Work out the finished part from the listing and answer in its coordinate system (mm). Face numbers are marked on the shaded views. A direction names the side the tool comes from. Give positions to 0.01 mm unless a question says otherwise; leave off trailing zeros. Write each loop counter-clockwise with the first axis right and the second up, starting at its lowest first coordinate (ties: lowest second). Pieces come first, ordered by that corner, then holes.
1) Given pin 1 Ø2 at (x, z) = (50, 44) entering from -Y; pin 2 Ø5 at (x, z) = (14, 6.5) entering from +Y; pin 3 Ø1.6 at (x, y) = (39, 110) entering from -Z; pin 4 Ø10 at (y, z) = (75.5, 37.5) entering from -X, each flat-ended and moving along its own axis, determine where each tip first touches the part or whether it passes through.
2) Find section A-A (y = 30). Determine the outline of the cut face in (x, z).
3) Find section B-B (x = 37). Count the separate pieces of the cut face and the enclosed holes in it, plus the area to 3 significant figures.
4) Determine the mould class of the marked faces 4, 5, 6 and 7 for opening direction Z: pulls with the +Z half, pulls with the -Z half, needs draft (parallel to the pull), parting line crosses it, or undercut.
5) A tool of negligible diameter and unlimited length cuts with its end or side. For the marked faces 1, 2 and 3, from which of +Z, -Z, +X, -X, +Y, -Y can it reach the whole face along a straight path? Write none if from no direction.
6) Straight lines are drawn through the part: probe 1 along Y at (x, z) = (55.5, 25.4); probe 2 along X at (y, z) = (11.5, 41); probe 3 along Z at (x, y) = (53, 107.5). For each, find the intervals that lie inside material, in ascending order.
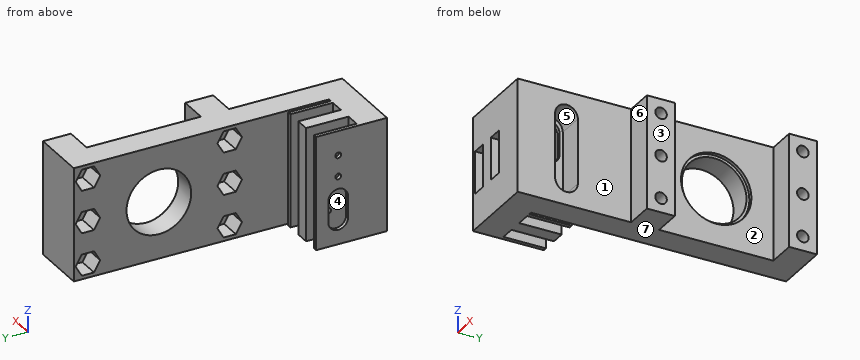
Autodesk Inventor part; units mm, degrees
ref_plane "YZ Plane" through (0, 0, 0) normal (1, 0, 0) x (0, 1, 0)
ref_plane "XZ Plane" through (0, 0, 0) normal (0, 1, 0) x (-1, 0, 0)
ref_plane "XY Plane" through (0, 0, 0) normal (0, 0, 1) x (1, 0, 0)
sketch "Sketch1" plane through (0, 0, 0) normal (0, 0, 1) x (1, 0, 0)
  line L0 (10.0241, 20.4474) -> (11.6941, 20.4474)
  line L1 (11.6941, 20.4474) -> (11.6941, -11.3026)
  line L2 (11.6941, -11.3026) -> (10.0241, -11.3026)
  line L3 (10.0241, -11.3026) -> (10.0241, 20.4474)
  line L4 (11.6941, -4.9526) -> (18.1941, -4.9526)
  line L5 (18.1941, -4.9526) -> (18.1941, -11.3026)
  line L6 (18.1941, -11.3026) -> (11.6941, -11.3026)
  line L7 (11.6941, -11.3026) -> (11.6941, -4.9526)
  line L8 (18.1941, 20.4474) -> (24.3941, 20.4474)
  line L9 (24.3941, 20.4474) -> (24.3941, -11.3026)
  line L10 (24.3941, -11.3026) -> (18.1941, -11.3026)
  line L11 (18.1941, -11.3026) -> (18.1941, 20.4474)
  line L12 (24.3941, -4.9526) -> (30.8941, -4.9526)
  line L13 (30.8941, -4.9526) -> (30.8941, -11.3026)
  line L14 (30.8941, -11.3026) -> (24.3941, -11.3026)
  line L15 (24.3941, -11.3026) -> (24.3941, -4.9526)
  line L16 (30.8941, 20.4474) -> (32.5641, 20.4474)
  line L17 (32.5641, 20.4474) -> (32.5641, -11.3026)
  line L18 (32.5641, -11.3026) -> (30.8941, -11.3026)
  line L19 (30.8941, -11.3026) -> (30.8941, 20.4474)
  line L20 (14.9441, -4.9526) -> (14.9441, -6.8027)
  line L21 (27.6441, -4.9526) -> (27.6441, -11.0357)
  line L22 (10.0241, 1.3974) -> (32.5641, 1.3974)
  line L23 (32.5641, 1.3974) -> (32.5641, -11.3026)
  line L24 (32.5641, -11.3026) -> (10.0241, -11.3026)
  line L25 (10.0241, -11.3026) -> (10.0241, 1.3974)
  line L26 (32.5641, -11.3026) -> (46.1861, -11.3026)
  line L27 (46.1861, -11.3026) -> (46.1861, 1.3974)
  line L28 (46.1861, 1.3974) -> (32.5641, 1.3974)
  line L29 (32.5641, 1.3974) -> (32.5641, -11.3026)
  line L30 (33.9941, 1.3974) -> (46.1861, 1.3974)
  line L31 (46.1861, 1.3974) -> (46.1861, 115.6974)
  line L32 (46.1861, 115.6974) -> (33.9941, 115.6974)
  line L33 (33.9941, 115.6974) -> (33.9941, 1.3974)
  line L34 (46.1861, 39.4974) -> (58.8861, 39.4974)
  line L35 (58.8861, 39.4974) -> (58.8861, 51.9974)
  line L36 (58.8861, 51.9974) -> (46.1861, 51.9974)
  line L37 (46.1861, 51.9974) -> (46.1861, 39.4974)
  line L38 (46.1861, 103.1974) -> (58.8861, 103.1974)
  line L39 (58.8861, 103.1974) -> (58.8861, 115.6974)
  line L40 (58.8861, 115.6974) -> (46.1861, 115.6974)
  line L41 (46.1861, 115.6974) -> (46.1861, 103.1974)
  line L42 (-51.3447, 77.5974) -> (150.8271, 77.5974) construction
  point P0 (0, 0)
  dimension "d0" = 6.5
  dimension "d1" = 6.5
  dimension "d4" = 12.7
  dimension "d5" = 1.67
  dimension "d6" = 25.4
  dimension "d51" = 12.5
  dimension "d52" = 12.5
  dimension "d53" = 51.2
  dimension "d54" = 57.15
  dimension "d55" = 25.6
  dimension "d57" = 12.7
  dimension "d58" = 12.192
  dimension "d59" = 18.542
  dimension "d60" = 12.7
  dimension "d86" = 76.2
  dimension "d114" = 76.2
extrude "Extrusion1" add sketch "Sketch1" along normal blind 50.8
sketch "Sketch9" plane through (46.1861, 51.9974, 0) normal (1, 0, 0) x (0, 0, -1)
  circle A0 centre (-25.4, 25.6) radius 15.7575
  line L0 (0, 0) -> (0, 51.2)
  line L1 (0, 51.2) -> (-50.8, 51.2)
  point P0 (0, -51.9974)
  dimension "d61" = 31.515
  dimension "d62" = 25.4
  dimension "d63" = 25.6
extrude "Extrusion8" cut sketch "Sketch9" against normal blind 1.651
sketch "Sketch10" plane through (44.5351, 77.5974, 25.4) normal (1, 0, 0) x (0, 0, -1)
  circle A0 centre (0, 0) radius 15.7575
  circle A1 centre (0, 0) radius 14.4875
  point P0 (25.4, -77.5974)
  dimension "d66" = 28.975
extrude "Extrusion9" cut sketch "Sketch10" against normal through all contours A1
sketch "Sketch11" plane through (10.0241, -11.3026, 0) normal (-1, 0, 0) x (0, 0, 1)
  circle A0 centre (25.4, 36.35) radius 2.25
  line L0 (0, 127) -> (0, 12.7)
  circle A1 centre (10.9, 21.85) radius 1.3
  circle A2 centre (20.4, 21.85) radius 1.3
  circle A3 centre (30.4, 21.85) radius 1.3
  circle A4 centre (39.9, 21.85) radius 1.3
  circle A5 centre (25.4, 88.9) radius 14.4875
  line L1 (36.7449, 38.6) -> (7.7398, 38.6) construction
  point P0 (0, 11.3026)
  dimension "d69" = 4.5
  dimension "d70" = 25.4
  dimension "d71" = 9.5
  dimension "d72" = 9.5
  dimension "d73" = 2.6
  dimension "d74" = 14.5
  dimension "d75" = 50.3
  dimension "d76" = 14.5
  dimension "d77" = 14.5
extrude "Extrusion10" cut sketch "Sketch11" against normal through all contours A1 | A2 | A3 | A4
sketch "Sketch14" plane through (30.8941, 1.3974, 0) normal (-1, 0, 0) x (0, 0, 1)
  circle A0 centre (39.9, 9.15) radius 1.3
  arc A1 (39.9, 4.705) -> (39.9, 13.595) centre (39.9, 9.15) ccw
  circle A2 centre (30.4, 9.15) radius 1.3
  arc A3 (30.4, 13.595) -> (30.4, 4.705) centre (30.4, 9.15) ccw
  line L0 (39.9, 4.705) -> (30.4, 4.705)
  line L1 (39.9, 13.595) -> (30.4, 13.595)
  arc A4 (39.9, 13.595) -> (39.9, 4.705) centre (39.9, 9.15) ccw
  arc A5 (30.4, 4.705) -> (30.4, 13.595) centre (30.4, 9.15) ccw
  point P0 (0, -1.3974)
  dimension "d87" = 8.89
extrude "Extrusion13" cut sketch "Sketch14" against normal up to surface (1.67 mm away)
sketch "Sketch15" plane through (10.0241, -11.3026, 0) normal (-1, 0, 0) x (0, 0, 1)
  circle A0 centre (20.4, 21.85) radius 1.3
  arc A1 (20.4, 17.405) -> (20.4, 26.295) centre (20.4, 21.85) ccw
  circle A2 centre (10.9, 21.85) radius 1.3
  arc A3 (10.9, 26.295) -> (10.9, 17.405) centre (10.9, 21.85) ccw
  line L0 (20.4, 17.405) -> (10.9, 17.405)
  line L1 (10.9, 26.295) -> (20.4, 26.295)
  arc A4 (20.4, 26.295) -> (20.4, 17.405) centre (20.4, 21.85) ccw
  arc A5 (10.9, 17.405) -> (10.9, 26.295) centre (10.9, 21.85) ccw
  point P0 (0, 11.3026)
  dimension "d90" = 8.89
extrude "Extrusion14" cut sketch "Sketch15" against normal up to surface (1.67 mm away)
sketch "Sketch16" plane through (46.1861, -11.3026, 0) normal (1, 0, 0) x (0, 0, -1)
  circle A0 centre (-10.9, 21.85) radius 1.3
  arc A1 (-10.9, 16.77) -> (-10.9, 26.93) centre (-10.9, 21.85) ccw
  circle A2 centre (-39.9, 21.85) radius 1.3
  arc A3 (-39.9, 26.93) -> (-39.9, 16.77) centre (-39.9, 21.85) ccw
  line L0 (-10.9, 16.77) -> (-39.9, 16.77)
  line L1 (-39.9, 26.93) -> (-10.9, 26.93)
  arc A4 (-10.9, 26.93) -> (-10.9, 16.77) centre (-10.9, 21.85) ccw
  arc A5 (-39.9, 16.77) -> (-39.9, 26.93) centre (-39.9, 21.85) ccw
  point P0 (0, 11.3026)
  dimension "d93" = 10.16
extrude "Extrusion15" cut sketch "Sketch16" against normal up to surface (12.192 mm away)
sketch "Sketch17" plane through (24.3941, 1.3974, 0) normal (0, 1, 0) x (1, 0, 0)
  line L0 (6.5, -34.925) -> (0, -34.925)
  line L1 (0, -34.925) -> (0, -15.875)
  line L2 (0, -15.875) -> (6.5, -15.875)
  line L3 (6.5, -15.875) -> (6.5, -34.925)
  line L4 (-6.2, -34.925) -> (-12.7, -34.925)
  line L5 (-12.7, -34.925) -> (-12.7, -15.875)
  line L6 (-12.7, -15.875) -> (-6.2, -15.875)
  line L7 (-6.2, -15.875) -> (-6.2, -34.925)
  line L8 (6.5, -25.4) -> (0, -25.4) construction
  line L9 (0, 0) -> (6.5, 0)
  line L10 (6.5, 0) -> (6.5, -50.8)
  line L11 (0, 0) -> (0, -50.8)
  line L12 (-6.2, 0) -> (-6.2, -50.8)
  line L13 (-12.7, 0) -> (-12.7, -50.8)
  point P0 (-24.3941, 0)
  dimension "d96" = 19.05
  dimension "d97" = 25.4
extrude "Extrusion16" cut sketch "Sketch17" against normal through all contours L0 L1 L2 L3 | L4 L5 L6 L7
sketch "Sketch19" plane through (58.8861, 39.4974, 0) normal (1, 0, 0) x (0, 0, -1)
  circle A0 centre (-6.35, 6.35) radius 2.5797
  line L0 (0, 12.5) -> (0, 63.7)
  line L1 (0, 0) -> (-50.8, 0)
  circle A1 centre (-6.35, 69.85) radius 2.5797
  circle A2 centre (-25.4, 6.35) radius 2.5797
  circle A3 centre (-25.4, 69.85) radius 2.5797
  circle A4 centre (-44.45, 6.35) radius 2.5797
  circle A5 centre (-44.45, 69.85) radius 2.5797
  circle A6 centre (-25.4, 38.1) radius 14.4875
  point P0 (0, -39.4974)
  dimension "d102" = 63.5
  dimension "d105" = 19.05
  dimension "d108" = 25.4
  dimension "d109" = 5.1594
  dimension "d110" = 31.75
extrude "Extrusion17" cut sketch "Sketch19" against normal through all contours A0 | A1 | A2 | A3 | A4 | A5
sketch "Sketch20" plane through (33.9941, 1.3974, 0) normal (-1, 0, 0) x (0, 0, 1)
  circle A0 centre (44.45, 107.95) radius 2.5797
  line L0 (49.2125, 105.2004) -> (44.45, 102.4507)
  line L1 (44.45, 102.4507) -> (39.6875, 105.2004)
  line L2 (39.6875, 105.2004) -> (39.6875, 110.6996)
  line L3 (39.6875, 110.6996) -> (44.45, 113.4493)
  line L4 (44.45, 113.4493) -> (49.2125, 110.6996)
  line L5 (49.2125, 110.6996) -> (49.2125, 105.2004)
  line L6 (0, 114.3) -> (50.8, 114.3)
  line L7 (50.8, 114.3) -> (50.8, 0)
  line L8 (30.1625, 105.2004) -> (25.4, 102.4507)
  line L9 (25.4, 102.4507) -> (20.6375, 105.2004)
  line L10 (20.6375, 105.2004) -> (20.6375, 110.6996)
  line L11 (20.6375, 110.6996) -> (25.4, 113.4493)
  line L12 (25.4, 113.4493) -> (30.1625, 110.6996)
  line L13 (30.1625, 110.6996) -> (30.1625, 105.2004)
  line L14 (11.1125, 105.2004) -> (6.35, 102.4507)
  line L15 (6.35, 102.4507) -> (1.5875, 105.2004)
  line L16 (1.5875, 105.2004) -> (1.5875, 110.6996)
  line L17 (1.5875, 110.6996) -> (6.35, 113.4493)
  line L18 (6.35, 113.4493) -> (11.1125, 110.6996)
  line L19 (11.1125, 110.6996) -> (11.1125, 105.2004)
  line L20 (49.2125, 41.7004) -> (44.45, 38.9507)
  line L21 (44.45, 38.9507) -> (39.6875, 41.7004)
  line L22 (39.6875, 41.7004) -> (39.6875, 47.1996)
  line L23 (39.6875, 47.1996) -> (44.45, 49.9493)
  line L24 (44.45, 49.9493) -> (49.2125, 47.1996)
  line L25 (49.2125, 47.1996) -> (49.2125, 41.7004)
  line L26 (30.1625, 41.7004) -> (25.4, 38.9507)
  line L27 (25.4, 38.9507) -> (20.6375, 41.7004)
  line L28 (20.6375, 41.7004) -> (20.6375, 47.1996)
  line L29 (20.6375, 47.1996) -> (25.4, 49.9493)
  line L30 (25.4, 49.9493) -> (30.1625, 47.1996)
  line L31 (30.1625, 47.1996) -> (30.1625, 41.7004)
  line L32 (11.1125, 41.7004) -> (6.35, 38.9507)
  line L33 (6.35, 38.9507) -> (1.5875, 41.7004)
  line L34 (1.5875, 41.7004) -> (1.5875, 47.1996)
  line L35 (1.5875, 47.1996) -> (6.35, 49.9493)
  line L36 (6.35, 49.9493) -> (11.1125, 47.1996)
  line L37 (11.1125, 47.1996) -> (11.1125, 41.7004)
  point P0 (0, -1.3974)
  point P1 (25.4, 107.95)
  point P2 (6.35, 107.95)
  point P3 (44.45, 44.45)
  point P4 (25.4, 44.45)
  point P5 (6.35, 44.45)
  dimension "d113" = 9.525
  dimension "d117" = 19.05
  dimension "d120" = 63.5
extrude "Extrusion18" cut sketch "Sketch20" against normal blind 9.525 contours A0 | L0 L1 L2 L3 L4 L5 | L8 L9 L10 L11 L12 L13 | L14 L15 L16 L17 L18 L19 | L20 L21 L22 L23 L24 L25 | L26 L27 L28 L29 L30 L31 | L32 L33 L34 L35 L36 L37
equation "\"d0\" = d1"
equation "\"d52\" = d51"
equation "\"d55\" = 0.5 * d53"
equation "\"d63\" = d55"
equation "\"d72\" = d71"
equation "\"d77\" = d76"
equation "\"d91\" = d90"
properties part number "RotateLimitSwitchHolder"
Results:
1. pin 1: stops at y = 39.5
1. pin 2: stops at y = 20.45
1. pin 3: stops at z = 0
1. pin 4: stops at x = 33.99
2. outline: (33.99, 0) - (46.19, 0) - (46.19, 50.8) - (33.99, 50.8) - close
3. separate pieces: 1
3. enclosed holes: 8
3. area: 4,950 mm2
4. face 4: undercut
4. face 5: undercut
4. face 6: needs draft
4. face 7: pulls with the -Z half
5. face 1: +Z, -Z, +X, -Y
5. face 2: +Z, -Z, +X
5. face 3: +Z, -Z, +X, +Y, -Y
6. probe 1: y = 39.5 to 43.27, 48.43 to 52, 103.2 to 106.77, 111.93 to 115.7
6. probe 2: x = 10.02 to 11.69, 18.19 to 24.39
6. probe 3: z = 0 to 4.55, 8.15 to 23.6, 27.2 to 42.65, 46.25 to 50.8
